Job drawing, mm, ordinate dimensions from the low corner. One solid piece. Give positions to 0.01 mm unless a question says otherwise; leave off trailing zeros. Write each loop counter-clockwise with the first axis right and the second up, starting at its lowest first coordinate (ties: lowest second). Pieces come first, ordered by that corner, then holes. Notation, with made-up numbers: (22, 82) - (34, 82) arc R18 ccw to (34, 97) - close; hole circle Ø1 at (-28, 58.5). An arc over 180 degrees is marked (long way). Put each result on its own line as item: value. Start each with the question number.
1. Cut at C-C on y = 2.05. List the corners of the cut face in (x, z).
2. Drop a flat-ended pin along its axis: pin 1 (1.8 mm diameter, centred on x = 148.75, z = 5, fed in from +Y). Give the stop position or say it passes through.
3. Wall check: line 1 (X direction, y = 2.9, z = 4.75); line 2 (Z direction, x = 166.25, y = 4); line 3 (X direction, y = 0.5, z = 4.25). Give the ranges that are in metal, low to high.
4. Cut at B-B on x = 130. List the corners of the cut face in (y, z), and give its area (3 significant figures).
5. Cut at A-A on z = 5. List the corners of the cut face in (x, y), and give its area (3 significant figures).
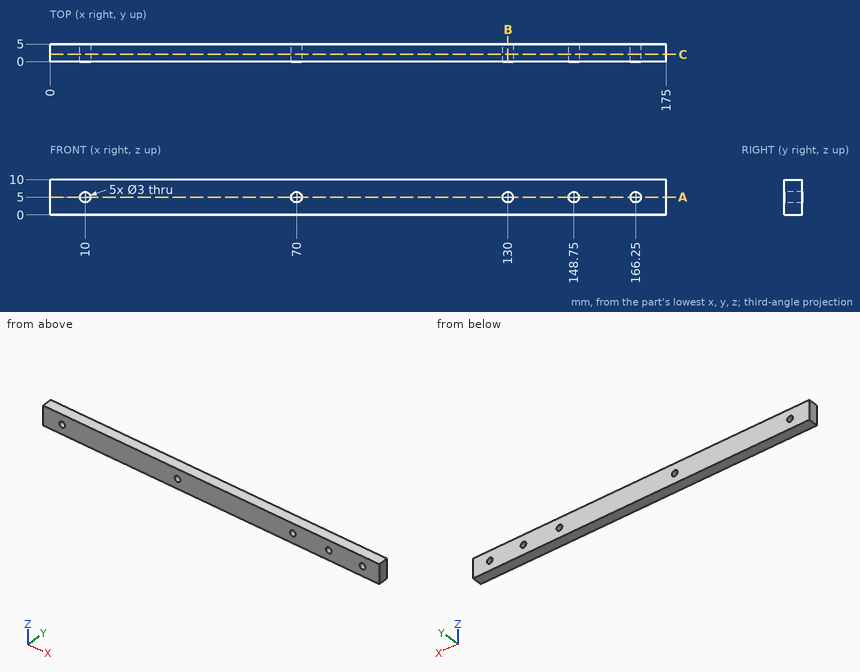
Report:
1. outline: (0, 0) - (175, 0) - (175, 10) - (0, 10) - close; hole circle Ø3 at (10, 5); hole circle Ø3 at (70, 5); hole circle Ø3 at (130, 5); hole circle Ø3 at (148.75, 5); hole circle Ø3 at (166.25, 5)
2. pin 1: passes through
3. line 1: x = 0 to 8.52, 11.48 to 68.52, 71.48 to 128.52, 131.48 to 147.27, 150.23 to 164.77, 167.73 to 175
3. line 2: z = 0 to 3.5, 6.5 to 10
3. line 3: x = 0 to 8.7, 11.3 to 68.7, 71.3 to 128.7, 131.3 to 147.45, 150.05 to 164.95, 167.55 to 175
4. outline: (0, 0) - (5, 0) - (5, 3.5) - (0, 3.5) - close; (0, 6.5) - (5, 6.5) - (5, 10) - (0, 10) - close
4. area: 35.0 mm²
5. outline: (0, 0) - (8.5, 0) - (8.5, 5) - (0, 5) - close; (11.5, 0) - (68.5, 0) - (68.5, 5) - (11.5, 5) - close; (71.5, 0) - (128.5, 0) - (128.5, 5) - (71.5, 5) - close; (131.5, 0) - (147.25, 0) - (147.25, 5) - (131.5, 5) - close; (150.25, 0) - (164.75, 0) - (164.75, 5) - (150.25, 5) - close; (167.75, 0) - (175, 0) - (175, 5) - (167.75, 5) - close
5. area: 800 mm²
